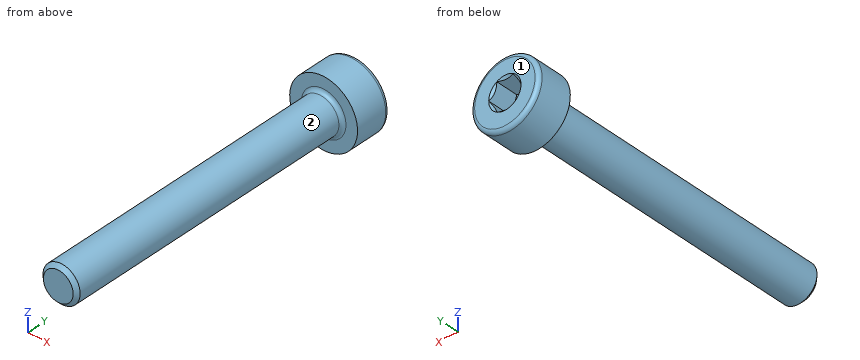
```python
from build123d import *

# Parameters (mm, degrees)
CUT_EXTRUDE1_DEPTH  = 1.1
BOSS_EXTRUDE1_REACH = 20.585
BOSS_EXTRUDE1_START = -0.5
SKETCH2_3_R         = 1.309481769


with BuildPart() as part:
    # Sketch1 → Revolve1 (revolve)
    with BuildSketch(Plane(origin=(0, 0, 0), x_dir=(0, 0, -1), z_dir=(1, 0, 0)), mode=Mode.PRIVATE) as revolve1_sk:
        with BuildLine():
            Line((0, -16), (0.8, -16))
            Line((0.8, -16), (1, -15.8))
            Line((1, -15.8), (1, -0.2))
            ThreePointArc((1, -0.2), (1.058578644, -0.058578644), (1.2, 0))
            Line((1.2, 0), (1.825, 0))
            Line((1.825, 0), (1.825, 1.7))
            ThreePointArc((1.825, 1.7), (1.766421356, 1.841421356), (1.625, 1.9))
            Line((1.625, 1.9), (0.8675, 1.9))
            Line((0.8675, 1.9), (0.75, 1.7825))
            Line((0.75, 1.7825), (0.75, 0.9))
            Line((0.75, 0.9), (0.8675, 0.9))
            Line((0.8675, 0.9), (0.8675, 0.7))
            Line((0.8675, 0.7), (0, 0.199148641))
            Line((0, 0.199148641), (0, -16))
        make_face()
    revolve(revolve1_sk.sketch.rotate(Axis((0, 2.837665271, 0), (0, -1, 0)), 180), axis=Axis((0, 2.837665271, 0), (0, -1, 0)))

    # Sketch2 → Cut-Extrude1 (cut)
    with BuildSketch(Plane(origin=(0, 1.9, 0), x_dir=(1, 0, 0), z_dir=(0, 1, 0))):
        Polygon((-0.866025404, 0), (-0.433012702, -0.75), (0.433012702, -0.75), (0.866025404, 0), (0.433012702, 0.75), (-0.433012702, 0.75), align=None)
    extrude(amount=-CUT_EXTRUDE1_DEPTH, mode=Mode.SUBTRACT)

    # Sketch2_3 → Boss-Extrude1 (add, up to next)
    with BuildSketch(Plane(origin=(0, 1.9, 0), x_dir=(1, 0, 0), z_dir=(0, 1, 0)).offset(BOSS_EXTRUDE1_START), mode=Mode.PRIVATE) as boss_extrude1_sk1:
        Circle(SKETCH2_3_R)
        Polygon((0.433012702, -0.75), (0.866025404, 0), (0.433012702, 0.75), (-0.433012702, 0.75), (-0.866025404, 0), (-0.433012702, -0.75), align=None, mode=Mode.SUBTRACT)
    boss_extrude1_tool1 = extrude(boss_extrude1_sk1.sketch, amount=-BOSS_EXTRUDE1_REACH, mode=Mode.PRIVATE) - part.part
    add(boss_extrude1_tool1.solids().sort_by_distance((-1.272444, 1.4, 0))[0])


solid = part.part
```
Geometry check sheet. Reference: the model listing, model coordinates, mm. Face numbers are marked on the shaded views. A direction names the side the tool comes from. Round coordinates to 2 decimals unless told otherwise and drop trailing zeros. Use a Markdown table: item, result.
Q1. Go/stop test with flat-tipped pins: P1, Ø1.1, axis at x = 1, z = -1, coming from the -Y side; P2, Ø1.5, axis at x = 0, y = -9.5, coming from the -Z side. Record where each tip stops, or that it passes through.
Solutions:
| item | result |
|---|---|
| P1 | stops at y = -15.94 |
| P2 | stops at z = -1 |
Q2. Material ranges on line 1 (Y direction, x = -0.8, z = 1.45); line 2 (X direction, y = -1.25, z = 0.9); line 3 (Z direction, x = 0.3, y = -1.75), recorded low to high.
Solutions:
| item | result |
|---|---|
| line 1 | y = 0 to 1.9 |
| line 2 | x = -0.44 to 0.44 |
| line 3 | z = -0.95 to 0.95 |
Q3. Access from +Z, -Z, +X, -X, +Y, -Y to the whole of each face (thin tool, end or side, straight path). Record for the marked faces 1 and 2.
Solutions:
| item | result |
|---|---|
| face 1 | +Z, -Z, +X, -X, +Y |
| face 2 | -Y |
